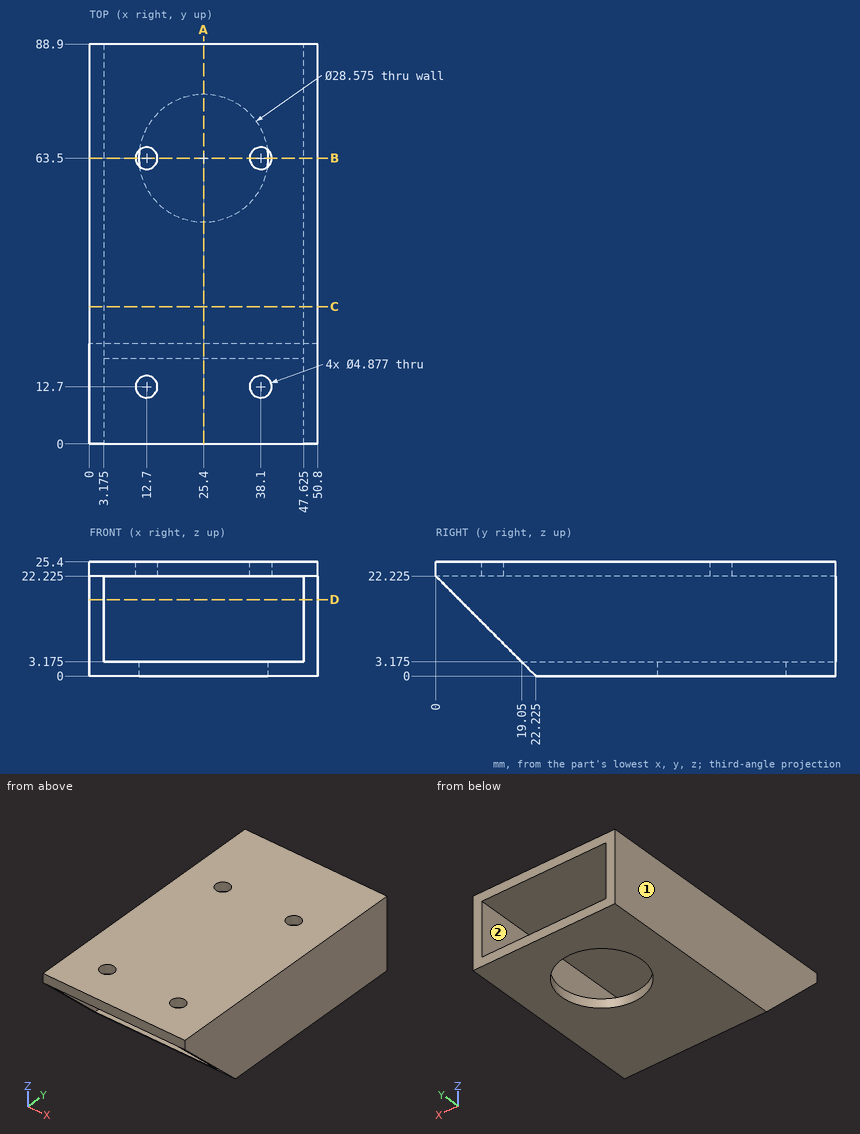
Can you work these out from the drawing? Everything is in mm from the part's minimum corner. A direction names the side the tool comes from. Coordinates: 2 decimals unless noted, no trailing zeros. Write each loop counter-clockwise with the first axis right and the second up, starting at its lowest first coordinate (ties: lowest second). Pieces come first, ordered by that corner, then holes. Notation, with made-up numbers: (57, -4.5) - (65, -4.5) arc R22 ccw to (65, 10.5) - close; hole circle Ø7 at (52.5, 87.5). An arc over 180 degrees is marked (long way). One line per item, written item: value.
1) Suppose I cut it at C-C on y = 30.5. Write out the boundary of the cut face in (x, z) (3 decimals).
Model answer:
outline: (0, 0) - (50.8, 0) - (50.8, 25.4) - (0, 25.4) - close; hole (3.175, 3.175) - (47.625, 3.175) - (47.625, 22.225) - (3.175, 22.225) - close
2) I'm going to push flat-ended pins straight in: P1, Ø5, axis at x = 37, z = 6, coming from the +Y side; P2, Ø6, axis at x = 17.5, y = 64, coming from the -Z side (3 decimals). Where does each tip first touch, or does it pass through?
Model answer:
P1: passes through
P2: stops at z = 22.225
3) I need wall thicknesses on line 1 along Y through (x, z) = (38.1, 24.6); line 2 along X through (y, z) = (32.5, 3.25) (3 decimals); line 3 along Z through (x, y) = (11, 73) (3 decimals). Which ranges of each line are inside material? Lowest first, please.
Model answer:
line 1: y = 0 to 10.26, 15.14 to 61.06, 65.94 to 88.9
line 2: x = 0 to 3.175, 47.625 to 50.8
line 3: z = 0 to 3.175, 22.225 to 25.4
4) Suppose I cut it at D-D on z = 17. Write out the boundary of the cut face in (x, y) (3 decimals).
Model answer:
outline: (0, 5.225) - (3.175, 5.225) - (3.175, 88.9) - (0, 88.9) - close; (47.625, 5.225) - (50.8, 5.225) - (50.8, 88.9) - (47.625, 88.9) - close
5) On a 3-axis mill with a long thin cutter (end or side, diameter ignored), from which of +Z, -Z, +X, -X, +Y, -Y can I reach the whole of each face in a straight line? I mean the marked faces 1 and 2. Say none if no direction works.
Model answer:
face 1: +Z, -Z, -X, +Y, -Y
face 2: +Y, -Y
6) Suppose I cut it at A-A on x = 25.4. State how many separate pieces and enclosed holes the cut face has, and give its area (3 significant figures).
Model answer:
separate pieces: 3
enclosed holes: 0
area: 408 mm²
7) Suppose I cut it at B-B on y = 63.5. Write out the boundary of the cut face in (x, z) (1 decimal).
Model answer:
outline: (0, 0) - (11.1, 0) - (11.1, 3.2) - (3.2, 3.2) - (3.2, 22.2) - (10.3, 22.2) - (10.3, 25.4) - (0, 25.4) - close; (15.1, 22.2) - (35.7, 22.2) - (35.7, 25.4) - (15.1, 25.4) - close; (39.7, 0) - (50.8, 0) - (50.8, 25.4) - (40.5, 25.4) - (40.5, 22.2) - (47.6, 22.2) - (47.6, 3.2) - (39.7, 3.2) - close
